Design review of the part built by this model. Coordinates are the model's own, in mm. A direction names the side the tool comes from. Coordinates: 2 decimals unless noted, no trailing zeros. Write each loop counter-clockwise with the first axis right and the second up, starting at its lowest first coordinate (ties: lowest second). Pieces come first, ordered by that corner, then holes. Notation, with made-up numbers: (25.5, -9) - (55.5, -9) arc R23 cw to (55.5, 17) - close; hole circle Ø10 at (39.25, 31). An arc over 180 degrees is marked (long way). One line per item, written item: value.
from build123d import *

# Parameters (mm, degrees)
BASE_DEPTH          = 3
SERVO_SUPPORT_DEPTH = 54.2
SERVO_MOUNTS_DEPTH  = 12.4
SERVO_SCREWS_REACH  = 146.657
SKETCH22_R          = 1.3
FILLET1_R           = 2
SKETCH23_W          = 12.651847812
SKETCH23_H          = 31.3
SHAFT_SUPPORT_DEPTH = 3
SKETCH24_W          = 5.5
SKETCH24_H          = 31.3
BOSS_EXTRUDE6_DEPTH = 66.6
FILLET2_R           = 8
FILLET3_R           = 8
SHAFT_REACH         = 152.69
SKETCH25_R          = 1.7
SCREWS_REACH        = 110.55
SKETCH26_R          = 1.6
SKETCH26_R_2        = 1.4
SKETCH31_W          = 7
SKETCH31_H          = 13.5765
BOSS_EXTRUDE8_DEPTH = 5
SKETCH30_R          = 2.5
BOSS_EXTRUDE9_DEPTH = 2.5
CUT_EXTRUDE1_REACH  = 125.131
SKETCH32_R          = 1.15
CHAMFER1_SIZE       = 2.5
CHAMFER2_SIZE       = 4


with BuildPart() as part:
    # Sketch19 → Base (new body)
    with BuildSketch(Plane.XY):
        Polygon((61.5, 19.3), (56.5, 19.3), (34, 29.3), (34, 34.3), (-59.5, 34.3), (-59.5, -43), (61.5, -43), align=None)
    extrude(amount=BASE_DEPTH)

    # Sketch20 → Servo support (add)
    with BuildSketch(Plane.XY):
        Polygon((-53.298152188, -10.85), (-55.448152188, -10.85), (-59.5, -10.85), (-59.5, 21.25), (-55.448152188, 21.25), (-53.298152188, 21.25), (-45.748152188, 21.25), (-45.748152188, 8.609473612), (-45.748152188, -10.85), align=None)
    extrude(amount=SERVO_SUPPORT_DEPTH)

    # Sketch21 → Servo mounts (add)
    with BuildSketch(Plane.XY.offset(54.2)):
        Polygon((-55.848152188, -6.2), (-59.5, -6.2), (-59.5, -10.85), (-55.648152188, -10.85), (-55.648152188, -6.2), align=None)
        Polygon((-55.848152188, 16.6), (-59.5, 16.6), (-59.5, 21.25), (-55.648152188, 21.25), (-55.648152188, 16.6), align=None)
    extrude(amount=SERVO_MOUNTS_DEPTH)

    # Sketch22 → Servo screws (cut, up to next)
    with BuildSketch(Plane.ZY.offset(59.5), mode=Mode.PRIVATE) as servo_screws_sk1:
        with Locations(Location((60.4, -8.65, 0), (0, 0, 270))):
            Circle(SKETCH22_R)
    servo_screws_tool1 = extrude(servo_screws_sk1.sketch, amount=-SERVO_SCREWS_REACH, mode=Mode.PRIVATE) & part.part
    # Sketch22 → Servo screws (cut, up to next)
    with BuildSketch(Plane.ZY.offset(59.5), mode=Mode.PRIVATE) as servo_screws_sk2:
        with Locations(Location((60.4, 19.05, 0), (0, 0, 270))):
            Circle(SKETCH22_R)
    servo_screws_tool2 = extrude(servo_screws_sk2.sketch, amount=-SERVO_SCREWS_REACH, mode=Mode.PRIVATE) & part.part
    add(servo_screws_tool1.solids().sort_by_distance((-59.5, -8.65, 60.4))[0], mode=Mode.SUBTRACT)
    add(servo_screws_tool2.solids().sort_by_distance((-59.5, 19.05, 60.4))[0], mode=Mode.SUBTRACT)

    # Fillet1
    fillet1_edges = [part.edges().sort_by_distance(p)[0] for p in [
        (-57.574076094, 21.25, 66.6),
        (-57.574076094, -10.85, 66.6),
    ]]
    fillet(fillet1_edges, radius=FILLET1_R)

    # Sketch23 → Shaft support (add)
    with BuildSketch(Plane.XY):
        with Locations((67.825923906, 3.65)):
            Rectangle(SKETCH23_W, SKETCH23_H)
    extrude(amount=SHAFT_SUPPORT_DEPTH)

    # Sketch24 → Boss-Extrude6 (add)
    with BuildSketch(Plane.XY):
        with Locations((71.401847812, 3.65)):
            Rectangle(SKETCH24_W, SKETCH24_H)
    extrude(amount=BOSS_EXTRUDE6_DEPTH)

    # Fillet2
    fillet2_edges = [part.edges().sort_by_distance(p)[0] for p in [
        (61.5, -12, 1.5),
    ]]
    fillet(fillet2_edges, radius=FILLET2_R)

    # Fillet3
    fillet3_edges = [part.edges().sort_by_distance(p)[0] for p in [
        (71.401847812, 19.3, 66.6),
        (71.825923906, -12, 66.6),
        (69.075325128, -12.011279749, 66.6),
    ]]
    fillet(fillet3_edges, radius=FILLET3_R)

    # Sketch25 → Shaft (cut, up to next)
    with BuildSketch(Plane.ZY.offset(-68.651847812), mode=Mode.PRIVATE) as shaft_sk1:
        with Locations((60.4, 0)):
            Circle(SKETCH25_R)
    shaft_tool1 = extrude(shaft_sk1.sketch, amount=-SHAFT_REACH, mode=Mode.PRIVATE) & part.part
    add(shaft_tool1.solids().sort_by_distance((68.651848, 0, 60.4))[0], mode=Mode.SUBTRACT)

    # Sketch26 → Screws (cut, up to next)
    with BuildSketch(Plane.XY, mode=Mode.PRIVATE) as screws_sk1:
        with Locations((-57, -40.5)):
            Circle(SKETCH26_R)
    screws_tool1 = extrude(screws_sk1.sketch, amount=SCREWS_REACH, mode=Mode.PRIVATE) & part.part
    # Sketch26 → Screws (cut, up to next)
    with BuildSketch(Plane.XY, mode=Mode.PRIVATE) as screws_sk2:
        with Locations((-10, -40.5)):
            Circle(SKETCH26_R)
    screws_tool2 = extrude(screws_sk2.sketch, amount=SCREWS_REACH, mode=Mode.PRIVATE) & part.part
    # Sketch26 → Screws (cut, up to next)
    with BuildSketch(Plane.XY, mode=Mode.PRIVATE) as screws_sk3:
        with Locations((59, -32)):
            Circle(SKETCH26_R)
    screws_tool3 = extrude(screws_sk3.sketch, amount=SCREWS_REACH, mode=Mode.PRIVATE) & part.part
    # Sketch26 → Screws (cut, up to next)
    with BuildSketch(Plane.XY, mode=Mode.PRIVATE) as screws_sk4:
        with Locations((59, 16.8)):
            Circle(SKETCH26_R)
    screws_tool4 = extrude(screws_sk4.sketch, amount=SCREWS_REACH, mode=Mode.PRIVATE) & part.part
    # Sketch26 → Screws (cut, up to next)
    with BuildSketch(Plane.XY, mode=Mode.PRIVATE) as screws_sk5:
        with Locations((31.5, 31.8)):
            Circle(SKETCH26_R)
    screws_tool5 = extrude(screws_sk5.sketch, amount=SCREWS_REACH, mode=Mode.PRIVATE) & part.part
    # Sketch26 → Screws (cut, up to next)
    with BuildSketch(Plane.XY, mode=Mode.PRIVATE) as screws_sk6:
        with Locations((-32.5, 31.8)):
            Circle(SKETCH26_R)
    screws_tool6 = extrude(screws_sk6.sketch, amount=SCREWS_REACH, mode=Mode.PRIVATE) & part.part
    # Sketch26 → Screws (cut, up to next)
    with BuildSketch(Plane.XY, mode=Mode.PRIVATE) as screws_sk7:
        with Locations((-57, 25.3)):
            Circle(SKETCH26_R)
    screws_tool7 = extrude(screws_sk7.sketch, amount=SCREWS_REACH, mode=Mode.PRIVATE) & part.part
    # Sketch26 → Screws (cut, up to next)
    with BuildSketch(Plane.XY, mode=Mode.PRIVATE) as screws_sk8:
        with Locations((-57, -14.5)):
            Circle(SKETCH26_R_2)
    screws_tool8 = extrude(screws_sk8.sketch, amount=SCREWS_REACH, mode=Mode.PRIVATE) & part.part
    # Sketch26 → Screws (cut, up to next)
    with BuildSketch(Plane.XY, mode=Mode.PRIVATE) as screws_sk9:
        with Locations((45.5, -40.5)):
            Circle(SKETCH26_R_2)
    screws_tool9 = extrude(screws_sk9.sketch, amount=SCREWS_REACH, mode=Mode.PRIVATE) & part.part
    add(screws_tool1.solids().sort_by_distance((-57, -40.5, 0))[0], mode=Mode.SUBTRACT)
    add(screws_tool2.solids().sort_by_distance((-10, -40.5, 0))[0], mode=Mode.SUBTRACT)
    add(screws_tool3.solids().sort_by_distance((59, -32, 0))[0], mode=Mode.SUBTRACT)
    add(screws_tool4.solids().sort_by_distance((59, 16.8, 0))[0], mode=Mode.SUBTRACT)
    add(screws_tool5.solids().sort_by_distance((31.5, 31.8, 0))[0], mode=Mode.SUBTRACT)
    add(screws_tool6.solids().sort_by_distance((-32.5, 31.8, 0))[0], mode=Mode.SUBTRACT)
    add(screws_tool7.solids().sort_by_distance((-57, 25.3, 0))[0], mode=Mode.SUBTRACT)
    add(screws_tool8.solids().sort_by_distance((-57, -14.5, 0))[0], mode=Mode.SUBTRACT)
    add(screws_tool9.solids().sort_by_distance((45.5, -40.5, 0))[0], mode=Mode.SUBTRACT)

    # Sketch31 → Boss-Extrude8 (add)
    with BuildSketch(Plane.XZ.offset(43)):
        with Locations((0, 9.78825)):
            Rectangle(SKETCH31_W, SKETCH31_H)
        with Locations((58, 9.78825)):
            Rectangle(SKETCH31_W, SKETCH31_H)
    extrude(amount=-BOSS_EXTRUDE8_DEPTH)

    # Sketch30 → Boss-Extrude9 (add)
    with BuildSketch(Plane.XZ.offset(43)):
        with Locations(Location((0, 13.0765, 0), (0, 0, 180))):
            Circle(SKETCH30_R)
        with Locations(Location((58, 13.0765, 0), (0, 0, 180))):
            Circle(SKETCH30_R)
    extrude(amount=BOSS_EXTRUDE9_DEPTH)

    # Sketch32 → Cut-Extrude1 (cut, up to next)
    with BuildSketch(Plane(origin=(0, -38, 0), x_dir=(1, 0, 0), z_dir=(0, 1, 0)), mode=Mode.PRIVATE) as cut_extrude1_sk1:
        with Locations(Location((0, -13.0765, 0), (0, 0, 270))):
            Circle(SKETCH32_R)
    cut_extrude1_tool1 = extrude(cut_extrude1_sk1.sketch, amount=-CUT_EXTRUDE1_REACH, mode=Mode.PRIVATE) & part.part
    # Sketch32 → Cut-Extrude1 (cut, up to next)
    with BuildSketch(Plane(origin=(0, -38, 0), x_dir=(1, 0, 0), z_dir=(0, 1, 0)), mode=Mode.PRIVATE) as cut_extrude1_sk2:
        with Locations(Location((58, -13.0765, 0), (0, 0, 270))):
            Circle(SKETCH32_R)
    cut_extrude1_tool2 = extrude(cut_extrude1_sk2.sketch, amount=-CUT_EXTRUDE1_REACH, mode=Mode.PRIVATE) & part.part
    add(cut_extrude1_tool1.solids().sort_by_distance((0, -38, 13.0765))[0], mode=Mode.SUBTRACT)
    add(cut_extrude1_tool2.solids().sort_by_distance((58, -38, 13.0765))[0], mode=Mode.SUBTRACT)

    # Chamfer1
    # the kernel refuses this chamfer: 2.5 mm, written as the material it adds along each edge
    with BuildSketch(Plane(origin=(58, -43, 13.0765), x_dir=(-1, 0, 0), z_dir=(0, 0, 1))) as chamfer1_piece_1_section:
        Polygon((2.5 + CHAMFER1_SIZE, 0), (2.5, CHAMFER1_SIZE), (2.5, 0), align=None)
    chamfer1_piece_1 = revolve(axis=Axis((58, -43, 13.0765), (0, -1, 0)), mode=Mode.PRIVATE)
    chamfer1_piece_1 = split(chamfer1_piece_1, bisect_by=Plane(origin=(61.5, -43.330528144, 9.079752975), z_dir=(-1, 0, 0)), keep=Keep.TOP, mode=Mode.PRIVATE)
    chamfer1_piece_1 = split(chamfer1_piece_1, bisect_by=Plane(origin=(54.5, -43.330528144, 9.079752975), z_dir=(1, 0, 0)), keep=Keep.TOP, mode=Mode.PRIVATE)
    chamfer1_piece_1 = split(chamfer1_piece_1, bisect_by=Plane(origin=(55.692477029, -43.330528144, 16.5765), z_dir=(0, 0, -1)), keep=Keep.TOP, mode=Mode.PRIVATE)
    chamfer1_piece_1 = split(chamfer1_piece_1, bisect_by=Plane(origin=(55.692477029, -45.5, 9.079752975), z_dir=(0, 1, 0)), keep=Keep.TOP, mode=Mode.PRIVATE)
    add(chamfer1_piece_1)
    with BuildSketch(Plane(origin=(0, -43, 13.0765), x_dir=(-1, 0, 0), z_dir=(0, 0, 1))) as chamfer1_piece_2_section:
        Polygon((2.5 + CHAMFER1_SIZE, 0), (2.5, CHAMFER1_SIZE), (2.5, 0), align=None)
    chamfer1_piece_2 = revolve(axis=Axis((0, -43, 13.0765), (0, -1, 0)), mode=Mode.PRIVATE)
    chamfer1_piece_2 = split(chamfer1_piece_2, bisect_by=Plane(origin=(-3.5, -43.330528144, 9.079752976), z_dir=(1, 0, 0)), keep=Keep.TOP, mode=Mode.PRIVATE)
    chamfer1_piece_2 = split(chamfer1_piece_2, bisect_by=Plane(origin=(-2.30752297, -43.330528144, 16.5765), z_dir=(0, 0, -1)), keep=Keep.TOP, mode=Mode.PRIVATE)
    chamfer1_piece_2 = split(chamfer1_piece_2, bisect_by=Plane(origin=(3.5, -43.330528144, 9.079752976), z_dir=(-1, 0, 0)), keep=Keep.TOP, mode=Mode.PRIVATE)
    chamfer1_piece_2 = split(chamfer1_piece_2, bisect_by=Plane(origin=(-2.30752297, -45.5, 9.079752976), z_dir=(0, 1, 0)), keep=Keep.TOP, mode=Mode.PRIVATE)
    add(chamfer1_piece_2)

    # Chamfer2
    chamfer2_edges = [part.edges().sort_by_distance(p)[0] for p in [
        (68.651847812, 3.627456407, 3),
    ]]
    chamfer(chamfer2_edges, length=CHAMFER2_SIZE)


solid = part.part
1. Mouldability with a two-part tool opening along X and no side actions: class faces 5 (the face through (-55.648, -8.6, 58.9)), 6 (the face through (34, 32, 1)), 7 (the face through (-1, -45.5, 14)) as released by +X, released by -X, zero draft, split by the parting line, or undercut.
Answer block:
face 5: undercut
face 6: released by +X
face 7: zero draft
2. For faces 1 (the face through (-53, 21.25, 33)), 2 (the face through (66.68, 3.06, 5.03)), 3 (the face through (69, 19.3, 22)), 4 (the face through (-58, -6.2, 60)), list the 3-axis set-ups (+Z, -Z, +X, -X, +Y, -Y) from which the entire face can be reached by the end or side of a thin tool; tool diameter is ignored.
Answer block:
face 1: +Z, +X, -X, +Y
face 2: +Z, +Y, -Y
face 3: +Z, -Z, +X, +Y
face 4: +Z, -X
3. Consider section B-B, the plane z = 56. Write out the cut boundary in (x, y), then the cut area to 3 significant figures.
Answer block:
outline: (-59.5, -10.85) - (-55.65, -10.85) - (-55.65, -6.2) - (-59.5, -6.2) - close; (-59.5, 16.6) - (-55.65, 16.6) - (-55.65, 21.25) - (-59.5, 21.25) - close; (68.65, -12.05) arc R8 cw to (69.5, -12) - (74.15, -12) - (74.15, 19.3) - (68.65, 19.3) - close
area: 208 mm^2
4. Wall thickness on line 1 along X through (y, z) = (-40.5, 1.7); line 2 along Y through (x, z) = (-57, 1); line 3 along X through (y, z) = (31.8, 0.9): over which ranges is each line inside the solid? List them lowest first.
Answer block:
line 1: x = -59.5 to -58.6, -55.4 to -11.6, -8.4 to 44.1, 46.9 to 61.5
line 2: y = -43 to -42.1, -38.9 to -15.9, -13.1 to 23.7, 26.9 to 34.3
line 3: x = -59.5 to -34.1, -30.9 to 29.9, 33.1 to 34
5. Insertion check: pin 1 Ø2 at (x, y) = (52, -34) entering from +Z; pin 2 Ø2 at (x, z) = (1, 12.5) entering from +Y; pin 3 Ø4 at (x, z) = (-57, 61) entering from -Y. Each pin has a flat end and moves straight along its axis. Give the tip position at first contact, or say it passes through.
Answer block:
pin 1: stops at z = 3
pin 2: stops at y = -38
pin 3: stops at y = -10.85
6. Consider section C-C, the plane y = -40.5. Write out the cut boundary in (x, z).
Answer block:
outline: (-59.5, 0) - (-58.6, 0) - (-58.6, 3) - (-59.5, 3) - close; (-55.4, 0) - (-11.6, 0) - (-11.6, 3) - (-55.4, 3) - close; (-8.4, 0) - (44.1, 0) - (44.1, 3) - (3.5, 3) - (3.5, 16.58) - (-3.5, 16.58) - (-3.5, 3) - (-8.4, 3) - close; (46.9, 0) - (61.5, 0) - (61.5, 16.58) - (54.5, 16.58) - (54.5, 3) - (46.9, 3) - close; hole circle Ø2.3 at (0, 13.08); hole circle Ø2.3 at (58, 13.08)
7. Consider section A-A, the plane y = 0. Write out the cut boundary in (x, z), then the cut area to 3 significant figures.
Answer block:
outline: (-59.5, 0) - (74.15, 0) - (74.15, 58.7) - (68.65, 58.7) - (68.65, 7) - (64.65, 3) - (-45.75, 3) - (-45.75, 54.2) - (-59.5, 54.2) - close; (68.65, 62.1) - (74.15, 62.1) - (74.15, 66.6) - (68.65, 66.6) - close
area: 1,440 mm^2
8. Consider section D-D, the plane x = 45.5. Write out the cut boundary in (y, z).
Answer block:
outline: (-43, 0) - (-41.9, 0) - (-41.9, 3) - (-43, 3) - close; (-39.1, 0) - (24.19, 0) - (24.19, 3) - (-39.1, 3) - close
